```python
from build123d import *

# Parameters (mm, degrees)
EXTRUDE_1_DEPTH     = 2
SKETCH_2_R          = 4.5
CUT_EXTRUDE_1_DEPTH = 139.507220028


with BuildPart() as part:
    # 草图1 → 凸台-拉伸1 (new body)
    with BuildSketch(Plane.XY):
        Polygon((-70, -20.5), (70, -20.5), (70, 20.5), (20.5, 20.5), (20.5, 119.5), (-20.5, 119.5), (-20.5, 20.5), (-70, 20.5), align=None)
    extrude(amount=EXTRUDE_1_DEPTH)

    # 草图2 → 切除-拉伸1 (cut, through all)
    with BuildSketch(Plane.XY.offset(2)):
        with Locations((0, 84.5)):
            Circle(SKETCH_2_R)
        with Locations((0, 44.5)):
            Circle(SKETCH_2_R)
        with Locations((-35, 0)):
            Circle(SKETCH_2_R)
        with Locations(Location((35, 0, 0), (0, 0, 180))):
            Circle(SKETCH_2_R)
    extrude(amount=-CUT_EXTRUDE_1_DEPTH, mode=Mode.SUBTRACT)


solid = part.part
```
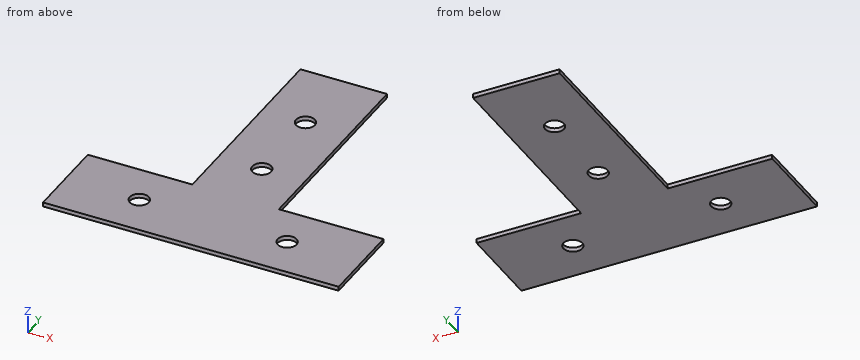
Here's how the part is built. I have some questions about the finished solid (model axes, mm). Round coordinates to 2 decimals unless told otherwise and drop trailing zeros. Order: outer loops, then holes, each group sorted by start corner. A loop starts at its lowest first (then second) coordinate and runs counter-clockwise, first axis right, second up. Notation, with made-up numbers: M 66,23.5 L 122,23.5 A26 cw 122,39.5 Z; hole C -11,-3.75 d5. An arc over 180 degrees is marked long. Answer in a Markdown table with one row per item.
Item 1: Imagine slicing it at A-A, the plane z = 1.6. Write out the boundary of the cut face in (x, y).
A:
| item | result |
|---|---|
| outline | M -70,-20.5 L 70,-20.5 L 70,20.5 L 20.5,20.5 L 20.5,119.5 L -20.5,119.5 L -20.5,20.5 L -70,20.5 Z; hole C -35,0 d9; hole C 0,44.5 d9; hole C 0,84.5 d9; hole C 35,0 d9 |
Item 2: If I drill on L1, parallel to X at y = 45, z = 0.65; L2, parallel to Y at x = 0, z = 1.15; L3, parallel to Y at x = 35, z = 1.35, over which ranges is the centre line in solid material (lowest first)? Write a range as from..to.
A:
| item | result |
|---|---|
| L1 | x = -20.5..-4.47, 4.47..20.5 |
| L2 | y = -20.5..40, 49..80, 89..119.5 |
| L3 | y = -20.5..-4.5, 4.5..20.5 |
Item 3: Imagine slicing it at B-B, the plane y = 0. Write out the boundary of the cut face in (x, z).
A:
| item | result |
|---|---|
| outline | M -70,0 L -39.5,0 L -39.5,2 L -70,2 Z; M -30.5,0 L 30.5,0 L 30.5,2 L -30.5,2 Z; M 39.5,0 L 70,0 L 70,2 L 39.5,2 Z |
Item 4: Imagine slicing it at D-D, the plane x = 0. Write out the boundary of the cut face in (y, z).
A:
| item | result |
|---|---|
| outline | M -20.5,0 L 40,0 L 40,2 L -20.5,2 Z; M 49,0 L 80,0 L 80,2 L 49,2 Z; M 89,0 L 119.5,0 L 119.5,2 L 89,2 Z |
Item 5: Imagine slicing it at C-C, the plane x = 35. Write out the boundary of the cut face in (y, z), and give its area (3 significant figures).
A:
| item | result |
|---|---|
| outline | M -20.5,0 L -4.5,0 L -4.5,2 L -20.5,2 Z; M 4.5,0 L 20.5,0 L 20.5,2 L 4.5,2 Z |
| area | 64.0 mm2 |
Item 6: I'm going to push flat-ended pins straight in: pin 1 (7 mm diameter, centred on x = -35, y = 0, fed in from -Z); pin 2 (1 mm diameter, centred on x = 44.5, z = 0.5, fed in from +Y); pin 3 (0.6 mm diameter, centred on y = 82.5, z = 1.5, fed in from +X). Where does each tip first touch, or does it pass through?
A:
| item | result |
|---|---|
| pin 1 | passes through |
| pin 2 | stops at y = 20.5 |
| pin 3 | stops at x = 20.5 |
